The model under review builds one solid part; all positions refer to its coordinate system, in mm. Face numbers are marked on the shaded views. Coordinates: 2 decimals unless noted, no trailing zeros. Write each loop counter-clockwise with the first axis right and the second up, starting at its lowest first coordinate (ties: lowest second). Pieces come first, ordered by that corner, then holes. Notation, with made-up numbers: M -22,58.5 L 2,58.5 A32 cw 2,86.5 Z; hole C 35,50.25 d3. An arc over 180 degrees is marked long. Answer as CSV lines item,"result". Start each with the question number.
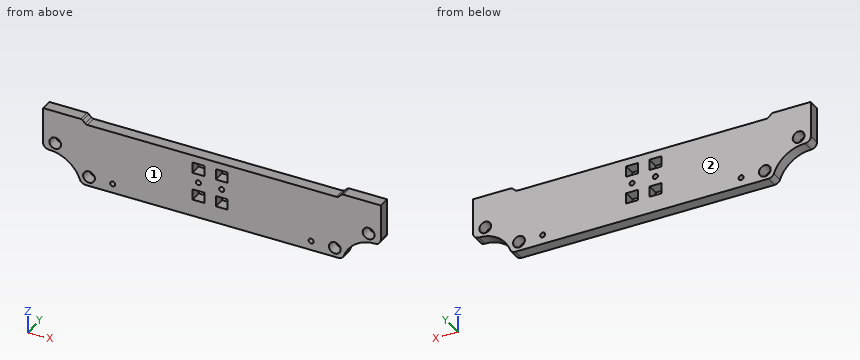
Autodesk Inventor part; units mm, degrees
ref_plane "Work Plane1" through (-117.5, 0, 47) normal (0, 0, 1) x (1, 0, 0)
ref_plane "YZ Plane" through (0, 0, 0) normal (1, 0, 0) x (0, 1, 0)
ref_plane "XY Plane" through (0, 0, 0) normal (0, 0, 1) x (1, 0, 0)
sketch "Sketch1" plane through (0, 0, 0) normal (0, 1, 0) x (-1, 0, 0)
  line L0 (-117.5, 47) -> (-117.5, 0)
  line L1 (-117.5, 0) -> (117.5, 0)
  line L2 (117.5, 0) -> (117.5, 47)
  line L3 (90.5, 47) -> (87.5, 44)
  line L4 (87.5, 44) -> (-87.5, 44)
  line L5 (-87.5, 44) -> (-90.5, 47)
  line L6 (117.5, 47) -> (90.5, 47)
  line L7 (-90.5, 47) -> (-117.5, 47)
  arc A0 (113.5, 18) -> (117.5, 22) centre (113.5, 22) ccw
  arc A1 (113.5, 18) -> (91, 0) centre (113.5, -5.0625) ccw
  line L8 (113.5, 22) -> (113.5, 18) construction
  arc A2 (-117.5, 22) -> (-113.5, 18) centre (-113.5, 22) ccw
  arc A3 (-91, 0) -> (-113.5, 18) centre (-113.5, -5.0625) ccw
  line L9 (-113.5, 22) -> (-113.5, 18) construction
  line L10 (0, 44) -> (0, 0) construction
  line L11 (13.5, 11.8) -> (5.3, 11.8)
  line L12 (5.3, 11.8) -> (5.3, 19.3)
  line L13 (5.3, 19.3) -> (13.5, 19.3)
  line L14 (13.5, 19.3) -> (13.5, 11.8)
  line L15 (13.5, 31.3) -> (5.3, 31.3)
  line L16 (5.3, 31.3) -> (5.3, 38.8)
  line L17 (5.3, 38.8) -> (13.5, 38.8)
  line L18 (13.5, 38.8) -> (13.5, 31.3)
  line L19 (-2.7, 11.8) -> (-10.9, 11.8)
  line L20 (-10.9, 11.8) -> (-10.9, 19.3)
  line L21 (-10.9, 19.3) -> (-2.7, 19.3)
  line L22 (-2.7, 19.3) -> (-2.7, 11.8)
  line L23 (-2.7, 31.3) -> (-10.9, 31.3)
  line L24 (-10.9, 31.3) -> (-10.9, 38.8)
  line L25 (-10.9, 38.8) -> (-2.7, 38.8)
  line L26 (-2.7, 38.8) -> (-2.7, 31.3)
  dimension "d1" = 235
  dimension "d2" = 3
  dimension "d3" = 45
  dimension "d4" = 27
  dimension "d5" = 47
  dimension "d6" = 4
  dimension "d7" = 29
  dimension "d8" = 23.0625
  dimension "d9" = 182
  dimension "d10" = 8.2
  dimension "d11" = 7.5
  dimension "d12" = 12
  dimension "d14" = 8
  dimension "d15" = 11.8
  dimension "d16" = 104
  dimension "d17" = 106.6
extrude "Extrusion1" add sketch "Sketch1" along normal blind 8 contours L7 L5 L4 L3 L6 L2 A0 A1 L1 A3 A2 L0
fillet "Fillet1" radius 4 2 edges at (-91, 4, 0) (91, 4, 0)
fillet "Fillet2" radius 2 4 edges at (-90.5, 4, 47) (-87.5, 4, 44) (87.5, 4, 44) (90.5, 4, 47)
sketch "Sketch2" plane through (0, 8, 0) normal (0, 1, 0) x (1, 0, 0)
  arc A0 (89.9142, -46.4142) -> (91.3284, -47) centre (91.3284, -45) ccw construction
  line L0 (91.3284, -47) -> (117.5, -47) construction
  line L1 (117.5, -47) -> (117.5, -22) construction
  arc A1 (117.5, -22) -> (113.5, -18) centre (113.5, -22) ccw construction
  arc A2 (91.7691, -2.6605) -> (113.5, -18) centre (113.5, 5.0625) ccw construction
  arc A3 (91.7691, -2.6605) -> (88, 0) centre (88, -4) ccw construction
  line L2 (88, 0) -> (-88, 0) construction
  arc A4 (-88, 0) -> (-91.7691, -2.6605) centre (-88, -4) ccw construction
  arc A5 (-113.5, -18) -> (-91.7691, -2.6605) centre (-113.5, 5.0625) ccw construction
  arc A6 (-113.5, -18) -> (-117.5, -22) centre (-113.5, -22) ccw construction
  line L3 (-117.5, -22) -> (-117.5, -47) construction
  line L4 (-117.5, -47) -> (-91.3284, -47) construction
  arc A7 (-91.3284, -47) -> (-89.9142, -46.4142) centre (-91.3284, -45) ccw construction
  line L5 (-89.9142, -46.4142) -> (-88.0858, -44.5858) construction
  arc A8 (-86.6716, -44) -> (-88.0858, -44.5858) centre (-86.6716, -46) ccw construction
  line L6 (-86.6716, -44) -> (86.6716, -44) construction
  arc A9 (88.0858, -44.5858) -> (86.6716, -44) centre (86.6716, -46) ccw construction
  line L7 (88.0858, -44.5858) -> (89.9142, -46.4142) construction
  line L8 (10.9, -31.3) -> (10.9, -38.8) construction
  line L9 (10.9, -38.8) -> (2.7, -38.8) construction
  line L10 (2.7, -38.8) -> (2.7, -31.3) construction
  line L11 (2.7, -31.3) -> (10.9, -31.3) construction
  line L12 (10.9, -11.8) -> (10.9, -19.3) construction
  line L13 (10.9, -19.3) -> (2.7, -19.3) construction
  line L14 (2.7, -19.3) -> (2.7, -11.8) construction
  line L15 (2.7, -11.8) -> (10.9, -11.8) construction
  line L16 (-5.3, -31.3) -> (-5.3, -38.8) construction
  line L17 (-5.3, -38.8) -> (-13.5, -38.8) construction
  line L18 (-13.5, -38.8) -> (-13.5, -31.3) construction
  line L19 (-13.5, -31.3) -> (-5.3, -31.3) construction
  line L20 (-5.3, -11.8) -> (-5.3, -19.3) construction
  line L21 (-5.3, -19.3) -> (-13.5, -19.3) construction
  line L22 (-13.5, -19.3) -> (-13.5, -11.8) construction
  line L23 (-13.5, -11.8) -> (-5.3, -11.8) construction
  line L24 (-13.5, -31.3) -> (-5.3, -31.3) construction
  line L25 (-9.4, -31.3) -> (-9.4, -19.3) construction
  line L26 (-5.3, -19.3) -> (-13.5, -19.3) construction
  line L27 (10.9, -31.3) -> (2.7, -31.3) construction
  line L28 (6.8, -31.3) -> (6.8, -19.3) construction
  point P0 (0, 0)
  point P1 (-9.4, -25.3)
  point P2 (6.8, -25.3)
  point P3 (-109, -24)
  point P4 (-85.5, -6.5)
  point P5 (-69, -6.5)
  point P6 (85.5, -6.5)
  point P7 (69, -6.5)
  point P8 (109, -24)
  dimension "d22" = 23
  dimension "d23" = 8.5
  dimension "d24" = 6.5
  dimension "d25" = 32
  dimension "d26" = 48.5
  dimension "d27" = 8.5
  dimension "d29" = 48.5
  dimension "d30" = 32
hole "Hole1" at (-9.4, 8, 25.3) at (6.8, 8, 25.3) at (-69, 8, 6.5) at (69, 8, 6.5) direction (0, -1, 0) diameter 3.5 end through all
hole "Hole2" at (-109, 8, 24) at (-85.5, 8, 6.5) at (85.5, 8, 6.5) at (109, 8, 24) direction (0, -1, 0) diameter 8.2 end through all
ref_plane "Work Plane1" through (-117.5, 0, 47) normal (0, 0, 1) x (1, 0, 0)
properties part number "A8-0008"
1) Take a section at B-B on y = 6.25. Give the number of separate pieces and of enclosed holes in the cut face, and give its area (3 significant figures).
2) Mouldability with a two-part tool opening along Y and no side actions: class the marked faces 1 and 2 as +Y half, -Y half, draft (parallel to the pull), parting line (faces both ways), or undercut.
3) To check wall thickness, follow line 1 (Z direction, x = 6.8, y = 3.5); line 2 (Z direction, x = -12, y = 1); line 3 (X direction, y = 4, z = 25.3). State the ranges of each line that lie inside material, in increasing order. Write a range as [from, to].
4) Take a section at C-C on x = 64.5. Give the boundary of the cut face in (y, z), and give its area (3 significant figures).
5) Take a section at A-A on x = 109. Give the boundary of the cut face in (y, z).
6) Clearance check with flat-ended pins moving along their axes: pin 1 Ø2 at (x, y) = (49, 4) entering from +Z; pin 2 Ø4 at (y, z) = (3.5, 17.5) entering from +X; pin 3 Ø4 at (y, z) = (5.5, 8.5) entering from +X. State where each tip first meets the part, or that it passes through.
Results:
1,separate pieces,"1"
1,enclosed holes,"12"
1,area,"9,260 mm²"
2,face 1,"-Y half"
2,face 2,"+Y half"
3,line 1,"z = [0, 11.8], [19.3, 23.55], [27.05, 31.3], [38.8, 44]"
3,line 2,"z = [0, 11.8], [19.3, 31.3], [38.8, 44]"
3,line 3,"x = [-117.5, -112.89], [-105.11, -11.15], [-7.65, 5.05], [8.55, 105.11], [112.89, 117.5]"
4,outline,"M 0,0 L 8,0 L 8,44 L 0,44 Z"
4,area,"352 mm²"
5,outline,"M 0,17.56 L 8,17.56 L 8,19.9 L 0,19.9 Z; M 0,28.1 L 8,28.1 L 8,47 L 0,47 Z"
6,pin 1,"stops at z = 44"
6,pin 2,"stops at x = 116.62"
6,pin 3,"stops at x = 96.48"
